Geometry check sheet. Reference: the model listing, model coordinates, mm. Face numbers are marked on the shaded views. A direction names the side the tool comes from. Coordinates: 2 decimals unless noted, no trailing zeros. Write each loop counter-clockwise with the first axis right and the second up, starting at its lowest first coordinate (ties: lowest second). Pieces come first, ordered by that corner, then holes. Notation, with made-up numbers: M -23.5,19 L 28.5,19 A15 cw 28.5,23 Z; hole C 57,54 d5. An arc over 180 degrees is marked long. Answer as a JSON object with one key per item and string values. Group by question number.
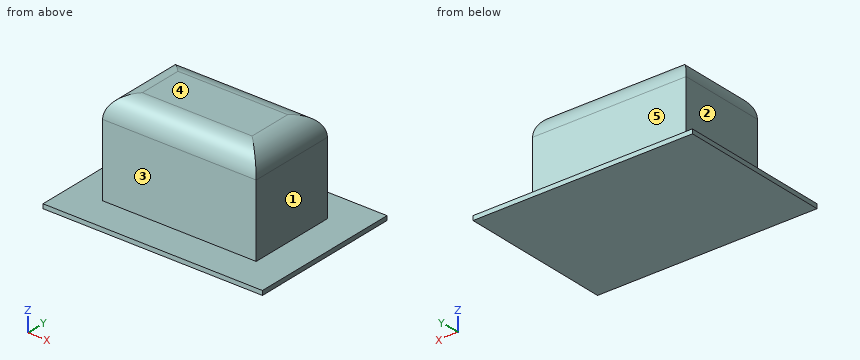
Autodesk Inventor part; units mm, degrees
ref_plane "YZ Plane" through (0, 0, 0) normal (1, 0, 0) x (0, 1, 0)
ref_plane "XZ Plane" through (0, 0, 0) normal (0, 1, 0) x (-1, 0, 0)
ref_plane "XY Plane" through (0, 0, 0) normal (0, 0, 1) x (1, 0, 0)
sketch "Sketch1" plane through (0, 0, 0) normal (0, 0, 1) x (1, 0, 0)
  line L0 (-1, 6) -> (9, 6)
  line L1 (9, 6) -> (9, -1)
  line L2 (9, -1) -> (-1, -1)
  line L3 (-1, -1) -> (-1, 6)
  line L4 (0.5, 4.5) -> (7.5, 4.5)
  line L5 (7.5, 4.5) -> (7.5, 0.5)
  line L6 (7.5, 0.5) -> (0.5, 0.5)
  line L7 (0.5, 0.5) -> (0.5, 4.5)
  point P0 (0, 0)
extrude "Extrusion1" add sketch "Sketch1" along normal blind 4.5 contours L0 L1 L2 L3 | L4 L5 L6 L7
sketch "Sketch2" plane through (0, 0, 4.5) normal (0, 0, 1) x (1, 0, 0)
  line L0 (-1, 6) -> (9, 6)
  line L1 (9, 6) -> (9, -1)
  line L2 (9, -1) -> (-1, -1)
  line L3 (-1, -1) -> (-1, 6)
  line L4 (0.5, 4.5) -> (7.5, 4.5)
  line L5 (7.5, 4.5) -> (7.5, 0.5)
  line L6 (7.5, 0.5) -> (0.5, 0.5)
  line L7 (0.5, 0.5) -> (0.5, 4.5)
  point P0 (0, 0)
  point P1 (0, 0)
extrude "Extrusion2" cut sketch "Sketch2" against normal blind 4.3
fillet "Fillet1" radius 1 4 edges at (0.5, 2.5, 4.5) (4, 0.5, 4.5) (7.5, 2.5, 4.5) (4, 4.5, 4.5)
properties part number "powerbutton"
1) Material ranges on probe 1 along X at (y, z) = (2, 0.7); probe 2 along Y at (x, z) = (6.25, 2.3); probe 3 along Z at (x, y) = (-0.25, 2), recorded low to high. Write a range as [from, to].
2) Go/stop test with flat-tipped pins: pin 1 Ø1.6 at (x, z) = (4, 1.5) entering from +Y; pin 2 Ø2 at (x, z) = (8, 2.5) entering from -Y. Record where each tip stops, or that it passes through.
3) Set-up check for the marked faces 1, 2, 3, 4 and 5: record each of +Z, -Z, +X, -X, +Y, -Y from which the full face is reachable in a straight line by a thin tool's end or side.
4) Section check B-B (x = 3.5). Record the cut outline in (y, z), then the cut area to 3 significant figures.
5) Section check A-A (y = 2.25). Record the cut outline in (x, z), then the cut area to 3 significant figures.
6) Section check C-C (z = 0.5). Record the cut outline in (x, y), then the cut area to 3 significant figures.
7) Section check D-D (x = 8). Record the cut outline in (y, z).
Entries:
{
 "1": {"probe 1": "[0.5, 7.5]", "probe 2": "[0.5, 4.5]", "probe 3": "[0, 0.2]"},
 "2": {"pin 1": "y = 4.5", "pin 2": "y = 0.5"},
 "3": {"face 1": "+Z, +X, +Y, -Y", "face 2": "+Z, -X, +Y, -Y", "face 3": "+Z, +X, -X, -Y", "face 4": "+Z, +X, -X, +Y, -Y", "face 5": "+Z, +X, -X, +Y"},
 "4": {"outline": "M -1,0 L 6,0 L 6,0.2 L 4.5,0.2 L 4.5,3.5 A1 ccw 3.5,4.5 L 1.5,4.5 A1 ccw 0.5,3.5 L 0.5,0.2 L -1,0.2 Z", "area": "18.2 mm^2"},
 "5": {"outline": "M -1,0 L 9,0 L 9,0.2 L 7.5,0.2 L 7.5,3.5 A1 ccw 6.5,4.5 L 1.5,4.5 A1 ccw 0.5,3.5 L 0.5,0.2 L -1,0.2 Z", "area": "31.7 mm^2"},
 "6": {"outline": "M 0.5,0.5 L 7.5,0.5 L 7.5,4.5 L 0.5,4.5 Z", "area": "28.0 mm^2"},
 "7": {"outline": "M -1,0 L 6,0 L 6,0.2 L -1,0.2 Z"}
}
